The model under review builds one solid part; all positions refer to its coordinate system, in mm. Face numbers are marked on the shaded views. Give positions to 0.01 mm unless a question says otherwise; leave off trailing zeros. Order: outer loops, then holes, each group sorted by start corner. A loop starts at its lowest first (then second) coordinate and runs counter-clockwise, first axis right, second up. Notation, with made-up numbers: (-21.5, 47.5) - (6.5, 47.5) arc R18 ccw to (6.5, 70.5) - close; hole circle Ø8 at (76.25, 71). An arc over 180 degrees is marked (long way). Put each result on its own line as item: value.
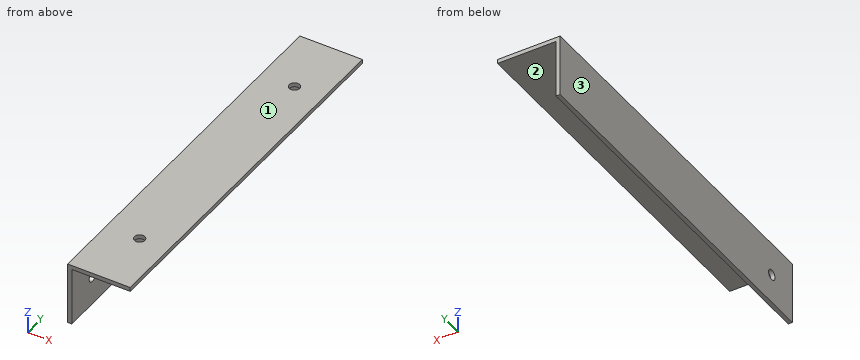
```python
from build123d import *

# Parameters (mm, degrees)
SKETCH_1_W      = 15
SKETCH_1_H      = 1
EXTRUDE_1_DEPTH = 90
SKETCH_3_W      = 1
SKETCH_3_H      = 90
EXTRUDE_2_DEPTH = 14
M3X0_5_1_D      = 2.5
M3X0_5_2_D      = 2.5


with BuildPart() as part:
    # ｽｹｯﾁ1 → ﾎﾞｽ - 押し出し1 (new body)
    with BuildSketch(Plane(origin=(0, 0, 0), x_dir=(1, 0, 0), z_dir=(0, 1, 0))):
        with Locations((7.5, -0.5)):
            Rectangle(SKETCH_1_W, SKETCH_1_H)
    extrude(amount=EXTRUDE_1_DEPTH)

    # ｽｹｯﾁ3 → ﾎﾞｽ - 押し出し2 (add)
    with BuildSketch(Plane(origin=(0, 0, 0), x_dir=(-1, 0, 0), z_dir=(0, 0, -1))):
        with Locations((-0.5, 45)):
            Rectangle(SKETCH_3_W, SKETCH_3_H)
    extrude(amount=EXTRUDE_2_DEPTH)

    # M3x0.5 ねじ穴1 (through all)
    with Locations(Plane.XY.offset(1)):
        with Locations((8, 15), (8, 75)):
            Hole(M3X0_5_1_D / 2)

    # M3x0.5 ねじ穴2 (through all)
    with Locations(Plane.ZY):
        with Locations((-7, 8)):
            Hole(M3X0_5_2_D / 2)


solid = part.part
```
(1) Wall thickness on L1, parallel to Y at x = 8, z = 0.8; L2, parallel to Y at x = 0.8, z = -7; L3, parallel to X at y = 75, z = 0.4: over which ranges is each line inside the solid? List them lowest first.
The answers:
L1: 0 to 13.75, 16.25 to 73.75, 76.25 to 90
L2: 0 to 6.75, 9.25 to 90
L3: 0 to 6.75, 9.25 to 15
(2) Take a section at C-C, the plane x = 7.75. Write out the cut boundary in (y, z), then the cut area to 3 significant figures.
The answers:
outline: (0, 0) - (13.78, 0) - (13.78, 1) - (0, 1) - close; (16.22, 0) - (73.78, 0) - (73.78, 1) - (16.22, 1) - close; (76.22, 0) - (90, 0) - (90, 1) - (76.22, 1) - close
area: 85.1 mm^2
(3) The part is to be moulded in two halves that separate along Z. For the marked faces 1, 2 and 3, say which applies: pulls with the +Z half, pulls with the -Z half, needs draft (parallel to the pull), parting line crosses it, or undercut.
The answers:
face 1: pulls with the +Z half
face 2: pulls with the -Z half
face 3: needs draft
(4) Take a section at B-B, the plane z = -7. Write out the cut boundary in (x, y).
The answers:
outline: (0, 0) - (1, 0) - (1, 6.75) - (0, 6.75) - close; (0, 9.25) - (1, 9.25) - (1, 90) - (0, 90) - close
(5) Clearance check with flat-ended pins moving along their axes: pin 1 Ø1.5 at (y, z) = (42, -5) entering from +X; pin 2 Ø2 at (x, z) = (11, -2.5) entering from +Y; pin 3 Ø6 at (x, y) = (12.5, 11) entering from -Z. State where each tip first meets the part, or that it passes through.
The answers:
pin 1: x = 1
pin 2: through
pin 3: z = 0
(6) Take a section at D-D, the plane y = 22.5. Write out the cut boundary in (x, z), then the cut area to 3 significant figures.
The answers:
outline: (0, -14) - (1, -14) - (1, 0) - (15, 0) - (15, 1) - (0, 1) - close
area: 29.0 mm^2
(7) Take a section at A-A, the plane y = 8. Write out the cut boundary in (x, z), then the cut area to 3 significant figures.
The answers:
outline: (0, -14) - (1, -14) - (1, -8.25) - (0, -8.25) - close; (0, -5.75) - (1, -5.75) - (1, 0) - (15, 0) - (15, 1) - (0, 1) - close
area: 26.5 mm^2
